from build123d import *

# Parameters (mm, degrees)
ESBO_O1_W                = 50
ESBO_O1_H                = 80
RESSALTO_EXTRUS_O1_DEPTH = 50
ESBO_O2_W                = 215
ESBO_O2_H                = 86
RESSALTO_EXTRUS_O2_DEPTH = 3
RESSALTO_EXTRUS_O3_DEPTH = 215


with BuildPart() as part:
    # Esboço1 → Ressalto-extrusão1 (new body)
    # profile 1 of 2: a face of its own
    with BuildSketch(Plane.XY):
        Polygon((53, 86), (0, 86), (0, 0), (53, 0), (56, 0), (56, 3), (56, 83), (56, 86), align=None)
        with Locations((28, 43)):
            Rectangle(ESBO_O1_W, ESBO_O1_H, mode=Mode.SUBTRACT)
    # profile 2 of 2: a face of its own
    with BuildSketch(Plane.XY):
        Polygon((215, 86), (56, 86), (56, 83), (106, 83), (106, 3), (56, 3), (56, 0), (215, 0), (215, 3), (215, 83), align=None)
        with Locations((134, 43)):
            Rectangle(ESBO_O1_W, ESBO_O1_H, mode=Mode.SUBTRACT)
        with Locations((187, 43)):
            Rectangle(ESBO_O1_W, ESBO_O1_H, mode=Mode.SUBTRACT)
    extrude(amount=RESSALTO_EXTRUS_O1_DEPTH)

    # Esboço2 → Ressalto-extrusão2 (add)
    with BuildSketch(Plane(origin=(0, 0, 0), x_dir=(-1, 0, 0), z_dir=(0, 0, -1))):
        with Locations((-107.5, 43)):
            Rectangle(ESBO_O2_W, ESBO_O2_H)
    extrude(amount=RESSALTO_EXTRUS_O2_DEPTH)

    # Esboço4 → Ressalto-extrusão3 (add)
    with BuildSketch(Plane(origin=(215, 0, 0), x_dir=(0, 0, -1), z_dir=(1, 0, 0))):
        Polygon((-59.230095943, 94), (-56.931962614, 95.928362829), (-48.601077026, 86), (-50, 86), (-50, 83), align=None)
    extrude(amount=-RESSALTO_EXTRUS_O3_DEPTH)


solid = part.part
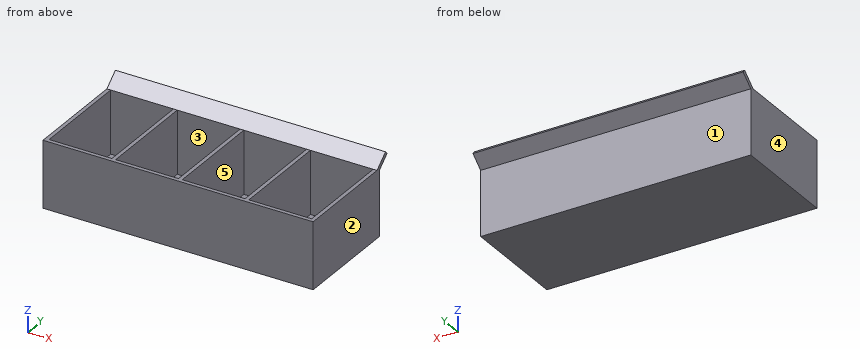
Input: part model. Units: mm. Frame: model coordinates. Face numbers are marked on the shaded views. A direction names the side the tool comes from. Coordinates: 2 decimals unless noted, no trailing zeros. Loops run counter-clockwise (first coordinate to the right, second up) from the corner with the lowest first, then second, coordinate; pieces in that order, holes last. Notation, with made-up numbers: (-9, 34) -> (50, 34) arc R36 ccw to (50, 73) -> close; hole circle Ø10 at (10, -26). An arc over 180 degrees is marked (long way). Write each question's results on one line, items separated by ' | '. Start each with the question number.
Q1. Pin query (flat end, axial travel): pin 1 (3 mm diameter, centred on y = 54.5, z = 50.5, fed in from +X); pin 2 (8 mm diameter, centred on x = 146.5, y = 65.5, fed in from +Z); pin 3 (12 mm diameter, centred on x = 105, y = 86, fed in from +Z). Return the tip coordinate at first contact, or that it passes through.
Q2. Section D-D, the plane z = 54.5. Return the cut outline in (x, y).
Q3. Ray query, line 1 (X direction, y = 50, z = 25.5); line 2 (Y direction, x = 19, z = 39.5); line 3 (Z direction, x = 31.5, y = 70). Return the intervals inside material, ascending. Write a range as from..to.
Q4. Reachability of the marked faces 4 and 5 from +Z, -Z, +X, -X, +Y, -Y: full face, straight path, thin tool, end or side. Return the list, or none.
Q5. Section C-C, the plane y = 63. Return the cut outline in (x, z).
Q6. Pull-direction query (Y, two-part tool) for the marked faces 1, 2 and 3; classes: released by +Y, released by -Y, zero draft, split by the parting line, or undercut.
Q7. Section B-B, the plane z = 18. Return the cut outline in (x, y).
Q8. Section A-A, the plane x = 64. Return the cut outline in (y, z).
Found:
1) pin 1: x = 215 | pin 2: z = 0 | pin 3: z = 57.55
2) outline: (0, 88.36) -> (215, 88.36) -> (215, 93.03) -> (0, 93.03) -> close
3) line 1: 0..3, 53..56, 106..109, 159..162, 212..215 | line 2: 0..3, 83..86 | line 3: -3..0
4) face 4: +Z, -Z, -X, +Y, -Y | face 5: +Z
5) outline: (0, -3) -> (215, -3) -> (215, 50) -> (212, 50) -> (212, 0) -> (162, 0) -> (162, 50) -> (159, 50) -> (159, 0) -> (109, 0) -> (109, 50) -> (106, 50) -> (106, 0) -> (56, 0) -> (56, 50) -> (53, 50) -> (53, 0) -> (3, 0) -> (3, 50) -> (0, 50) -> close
6) face 1: released by +Y | face 2: zero draft | face 3: undercut
7) outline: (0, 0) -> (215, 0) -> (215, 86) -> (0, 86) -> close; hole (3, 3) -> (53, 3) -> (53, 83) -> (3, 83) -> close; hole (56, 3) -> (106, 3) -> (106, 83) -> (56, 83) -> close; hole (109, 3) -> (159, 3) -> (159, 83) -> (109, 83) -> close; hole (162, 3) -> (212, 3) -> (212, 83) -> (162, 83) -> close
8) outline: (0, -3) -> (86, -3) -> (86, 48.6) -> (95.93, 56.93) -> (94, 59.23) -> (83, 50) -> (83, 0) -> (3, 0) -> (3, 50) -> (0, 50) -> close
